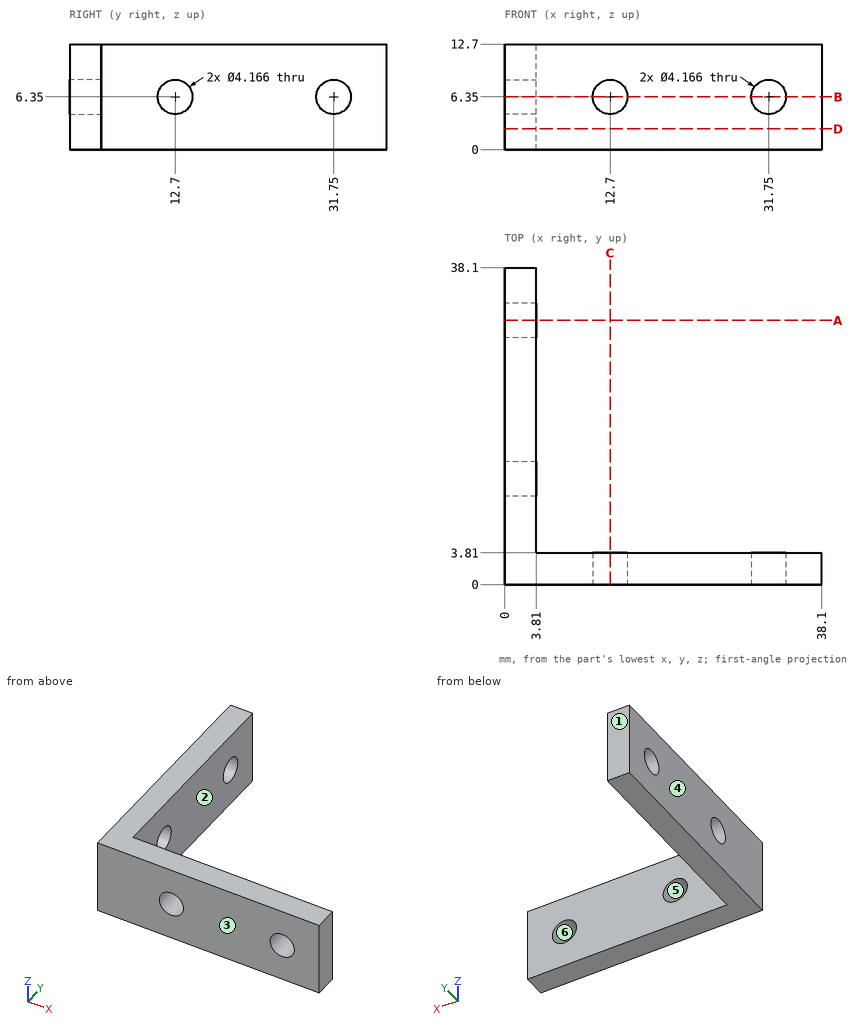
Study the drawing (mm; zero at the part's minimum x, y, z) and answer. A direction names the side the tool comes from. Round coordinates to 2 decimals unless told otherwise and drop trailing zeros. Write each loop counter-clockwise with the first axis right and the second up, starting at its lowest first coordinate (ties: lowest second). Pieces come first, ordered by that corner, then holes.
1) A cutting plane is placed at A-A on y = 31.75. Determine the outline of the cut face in (x, z), and give its area (3 significant figures).
2) Flat-ended cylindrical pins translate along their axes: P1, Ø1, axis at y = 4, z = 6, coming from the +X side; P2, Ø6.5, axis at x = 29, z = 7, coming from the +Y side; P3, Ø5.5, axis at y = 12.7, z = 6.35, coming from the +X side. Find the tip coordinate at first contact, or state that the pin passes through.
3) Determine the mould class of the marked faces 3, 4, 5 and 6 for opening direction X: pulls with the +X half, pulls with the -X half, needs draft (parallel to the pull), parting line crosses it, or undercut.
4) Consider probe 1 along Y at (x, z) = (2.5, 6.35); probe 2 along Z at (x, y) = (12.7, 2.5). Determine where each line is inside the solid, lowest interval first.
5) Which of the six approach directions +Z, -Z, +X, -X, +Y, -Y give full straight-line access (tool end or side, diameter ignored) to the marked faces 1 and 2?
6) A cutting plane is placed at D-D on z = 2.5. Determine the outline of the cut face in (x, y).
7) A cutting plane is placed at B-B on z = 6.35. Determine the outline of the cut face in (x, y), and give its area (3 significant figures).
Entries:
1. outline: (0, 0) - (3.81, 0) - (3.81, 4.27) - (0, 4.27) - close; (0, 8.43) - (3.81, 8.43) - (3.81, 12.7) - (0, 12.7) - close
1. area: 32.5 mm2
2. P1: stops at x = 38.1
2. P2: stops at y = 3.81
2. P3: stops at x = 3.81
3. face 3: needs draft
3. face 4: pulls with the -X half
3. face 5: undercut
3. face 6: undercut
4. probe 1: y = 0 to 10.62, 14.78 to 29.67, 33.83 to 38.1
4. probe 2: z = 0 to 4.27, 8.43 to 12.7
5. face 1: +Z, -Z, +X, -X, +Y
5. face 2: +Z, -Z, +X, +Y
6. outline: (0, 0) - (38.1, 0) - (38.1, 3.81) - (3.81, 3.81) - (3.81, 38.1) - (0, 38.1) - close
7. outline: (0, 0) - (10.62, 0) - (10.62, 3.81) - (3.81, 3.81) - (3.81, 10.62) - (0, 10.62) - close; (0, 14.78) - (3.81, 14.78) - (3.81, 29.67) - (0, 29.67) - close; (0, 33.83) - (3.81, 33.83) - (3.81, 38.1) - (0, 38.1) - close; (14.78, 0) - (29.67, 0) - (29.67, 3.81) - (14.78, 3.81) - close; (33.83, 0) - (38.1, 0) - (38.1, 3.81) - (33.83, 3.81) - close
7. area: 212 mm2
